Job drawing, mm, ordinate dimensions from the low corner. One solid piece. A direction names the side the tool comes from. Give positions to 0.01 mm unless a question says otherwise; leave off trailing zeros. Order: outer loops, then holes, each group sorted by start corner. A loop starts at its lowest first (then second) coordinate and runs counter-clockwise, first axis right, second up. Notation, with made-up numbers: (17.5, 56) - (76.5, 56) arc R10 ccw to (76.5, 75) - close; hole circle Ø6 at (-30.5, -22). An arc over 180 degrees is marked (long way). One line per item, written item: value.
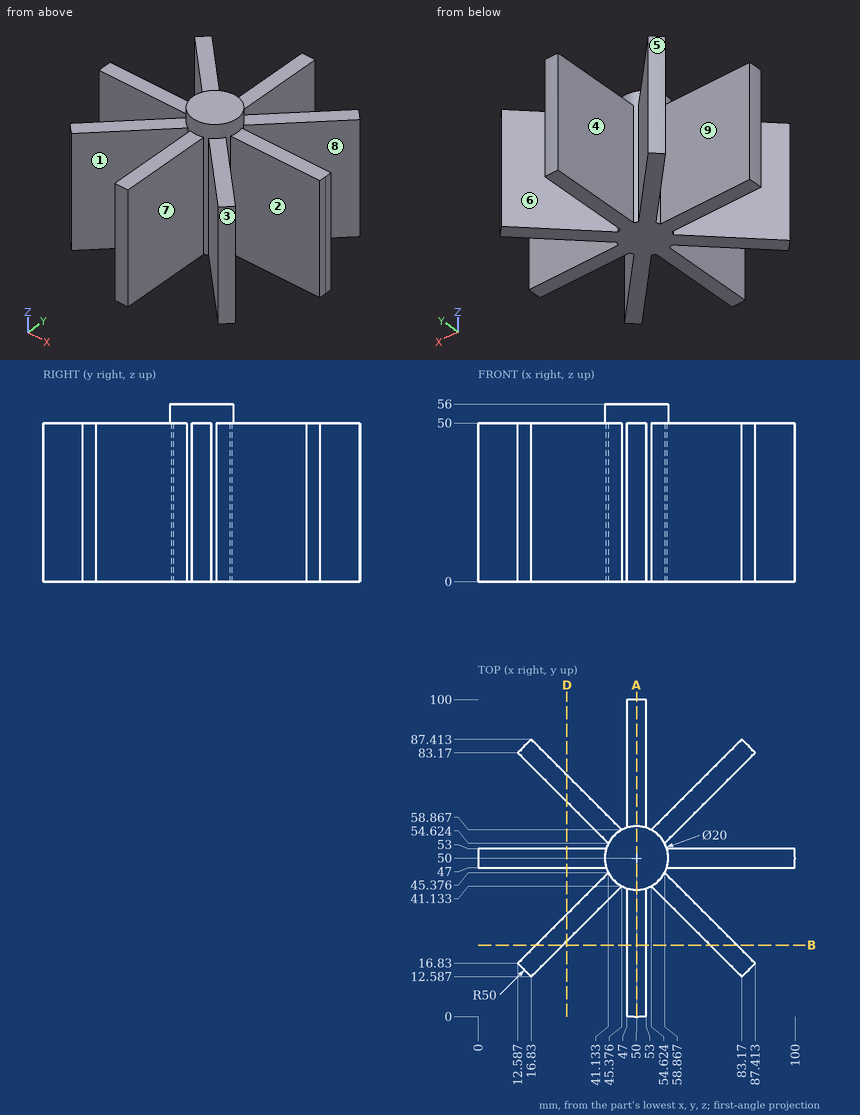
1) Two-plate mould, pull along X, no slides. Class the marked faces 1, 2, 3 and 4: pulls with the +X half, pulls with the -X half, needs draft (parallel to the pull), parting line crosses it, or undercut.
Answer:
face 1: undercut
face 2: needs draft
face 3: pulls with the +X half
face 4: undercut
2) Slice it at B-B on y = 22.5. Write the cut outline in (x, z).
Answer:
outline: (18.26, 0) - (26.74, 0) - (26.74, 50) - (18.26, 50) - close; (47, 0) - (53, 0) - (53, 50) - (47, 50) - close; (73.26, 0) - (81.74, 0) - (81.74, 50) - (73.26, 50) - close
3) Slice it at A-A on x = 50. Write the cut outline in (y, z), then the cut area to 3 significant figures.
Answer:
outline: (0, 0) - (100, 0) - (100, 50) - (60, 50) - (60, 56) - (40, 56) - (40, 50) - (0, 50) - close
area: 5,120 mm2
4) Drop flat-ended pins along their axis: P1, Ø12, axis at y = 15, z = 32, coming from the -X side; P2, Ø8, axis at x = 71.5, z = 41.5, coming from the -Y side; P3, Ø3, axis at y = 28.5, z = 32.5, coming from the -X side. Give the stop position or say it passes through.
Answer:
P1: stops at x = 12.59
P2: stops at y = 20.26
P3: stops at x = 22.76
5) Wall check: line 1 along Y through (x, z) = (25, 11.5); line 2 along X through (y, z) = (73, 18.5); line 3 along X through (y, z) = (21, 40.5). Give the ranges that are in metal, low to high. Write a range as [from, to].
Answer:
line 1: y = [20.76, 29.24], [47, 53], [70.76, 79.24]
line 2: x = [22.76, 31.24], [47, 53], [68.76, 77.24]
line 3: x = [16.76, 25.24], [47, 53], [74.76, 83.24]
6) Which spindle directions (+Z, -Z, +X, -X, +Y, -Y) get a long thin tool onto all of the face, cutting with end or side? Do the marked faces 5, 6, 7, 8 and 9. Say none if no direction does.
Answer:
face 5: +Z, -Z, -X, +Y
face 6: +Z, -Z, +Y
face 7: +Z, -Z, -Y
face 8: +Z, -Z, +X
face 9: +Z, -Z, -X
7) Slice it at D-D on x = 28. Write the cut outline in (y, z), then the cut area to 3 significant figures.
Answer:
outline: (23.76, 0) - (32.24, 0) - (32.24, 50) - (23.76, 50) - close; (47, 0) - (53, 0) - (53, 50) - (47, 50) - close; (67.76, 0) - (76.24, 0) - (76.24, 50) - (67.76, 50) - close
area: 1,150 mm2
